For this review, take the finished solid that the model builds, in its own axes (mm). A direction names the side the tool comes from. Round coordinates to 2 decimals unless told otherwise and drop trailing zeros. Write each loop counter-clockwise with the first axis right and the second up, starting at its lowest first coordinate (ties: lowest second). Pieces come first, ordered by that corner, then holes. Notation, with made-up numbers: M 56.25,78 L 83.25,78 A23 cw 83.25,113 Z; hole C 31.25,24 d8. An arc over 180 degrees is marked long. Answer in a Markdown table with one row per item.
Autodesk Fusion 360 part; units mm, degrees
sketch "Sketch1" plane through (0, 0, 0) normal (0, 0, 1) x (1, 0, 0)
  line L0 (0, 0) -> (120, 0)
  line L1 (120, 0) -> (120, 50)
  line L2 (120, 50) -> (0, 50)
  line L3 (0, 50) -> (0, 0)
  line L4 (16.75, 41.3333) -> (103.25, 41.3333)
  line L5 (103.25, 41.3333) -> (103.25, 29.3333)
  line L6 (103.25, 29.3333) -> (16.75, 29.3333)
  line L7 (16.75, 29.3333) -> (16.75, 41.3333)
  line L8 (16.75, 20.6667) -> (103.25, 20.6667)
  line L9 (103.25, 20.6667) -> (103.25, 8.6667)
  line L10 (103.25, 8.6667) -> (16.75, 8.6667)
  line L11 (16.75, 8.6667) -> (16.75, 20.6667)
  line L12 (103.25, 35.3656) -> (120, 35.3656) construction
  line L13 (0, 36) -> (16.75, 36) construction
  line L14 (16.75, 14.6667) -> (0, 14.6667) construction
  line L15 (103.25, 14.6667) -> (120, 14.6667) construction
  line L16 (54.6731, 50) -> (54.6731, 41.3333) construction
  line L17 (54.6731, 29.3333) -> (54.6731, 20.6667) construction
  line L18 (56.6135, 8.6667) -> (56.6135, 0) construction
  dimension "d1" = 120
  dimension "d2" = 50
  dimension "d3" = 86.5
  dimension "d4" = 12
  dimension "d6" = 86.5
  dimension "d7" = 12
extrude "Extrude1" add sketch "Sketch1" along normal blind 2
sketch "Sketch2" plane through (0, 0, 2) normal (0, 0, 1) x (-1, 0, 0)
  line L0 (-103.25, -8.6667) -> (-16.75, -8.6667)
  line L1 (-16.75, -8.6667) -> (-16.75, -20.6667)
  line L2 (-16.75, -20.6667) -> (-103.25, -20.6667)
  line L3 (-103.25, -20.6667) -> (-103.25, -8.6667)
  line L4 (-103.25, -29.3333) -> (-16.75, -29.3333)
  line L5 (-16.75, -29.3333) -> (-16.75, -41.3333)
  line L6 (-16.75, -41.3333) -> (-103.25, -41.3333)
  line L7 (-103.25, -41.3333) -> (-103.25, -29.3333)
  line L8 (0, -50) -> (0, 0)
  line L9 (0, 0) -> (-120, 0)
  line L10 (-120, 0) -> (-120, -50)
  line L11 (-120, -50) -> (0, -50)
  line L12 (-2, -48) -> (-118, -48)
  line L13 (-118, -48) -> (-118, -2)
  line L14 (-118, -2) -> (-2, -2)
  line L15 (-2, -2) -> (-2, -48)
  dimension "d10" = 2
  dimension "d11" = 2
  dimension "d12" = 2
  dimension "d13" = 2
extrude "Extrude2" add sketch "Sketch2" along normal blind 50 contours L8 L9 L10 L11
sketch "Sketch3" plane through (0, 0, 0) normal (-1, 0, 0) x (0, -1, 0)
  line L0 (-50, 0) -> (0, 0)
  line L1 (0, 0) -> (0, 52)
  line L2 (0, 52) -> (-50, 52)
  line L3 (-50, 52) -> (-50, 0)
  line L4 (-31, 47) -> (-19, 47)
  line L5 (-19, 47) -> (-19, 42)
  line L6 (-19, 42) -> (-31, 42)
  line L7 (-31, 42) -> (-31, 47)
  line L8 (-31, 44.5) -> (-50, 44.5) construction
  line L9 (-40.8681, 44.5) -> (-40.5, 44.5) construction
  line L10 (-19, 44.5) -> (0, 44.5) construction
  dimension "d16" = 12
  dimension "d17" = 5
  dimension "d18" = 5
extrude "Extrude3" cut sketch "Sketch3" against normal blind 10 contours L4 L5 L6 L7
Q1. Take a section at C-C (z = 32.5). State the section outline as (x, y) points.
Found:
| item | result |
|---|---|
| outline | M 0,0 L 120,0 L 120,50 L 0,50 Z; hole M 2,2 L 118,2 L 118,48 L 2,48 Z |
Q2. Take a section at D-D (z = 45). State the section outline as (x, y) points, then the cut area to 3 significant figures.
Found:
| item | result |
|---|---|
| outline | M 0,0 L 120,0 L 120,50 L 0,50 L 0,31 L 2,31 L 2,48 L 118,48 L 118,2 L 2,2 L 2,19 L 0,19 Z |
| area | 640 mm² |
Q3. Take a section at B-B (y = 34.5). State the section outline as (x, z) points, then the cut area to 3 significant figures.
Found:
| item | result |
|---|---|
| outline | M 0,0 L 16.75,0 L 16.75,2 L 2,2 L 2,52 L 0,52 Z; M 103.25,0 L 120,0 L 120,52 L 118,52 L 118,2 L 103.25,2 Z |
| area | 267 mm² |
Q4. For probe 1 along X at (y, z) = (14.5, 22); probe 2 along Y at (x, z) = (93.5, 8); probe 3 along Z at (x, y) = (8, 38), list the stretches that pass through material, from the lowest coordinate up.
Found:
| item | result |
|---|---|
| probe 1 | 0 to 2, 118 to 120 |
| probe 2 | 0 to 2, 48 to 50 |
| probe 3 | 0 to 2 |
Q5. Machinability: for faces 4 (the face through (2, 25, 27)), 5 (the face through (61, 50, 26)), which of the approach directions +Z, -Z, +X, -X, +Y, -Y give a long, thin tool a straight path to every point of the face, cutting with its end or side? Answer none if there is none.
Found:
| item | result |
|---|---|
| face 4 | +Z |
| face 5 | +Z, -Z, +X, -X, +Y |
Q6. Mouldability with a two-part tool opening along X and no side actions: class faces 1 (the face through (59, 25, 0)), 2 (the face through (61, 2, 27)), 3 (the face through (120, 25, 26)) as +X half, -X half, draft (parallel to the pull), parting line (faces both ways), or undercut.
Found:
| item | result |
|---|---|
| face 1 | draft |
| face 2 | undercut |
| face 3 | +X half |
Q7. Take a section at A-A (x = 76.5). State the section outline as (y, z) points, then the cut area to 3 significant figures.
Found:
| item | result |
|---|---|
| outline | M 0,0 L 8.67,0 L 8.67,2 L 2,2 L 2,52 L 0,52 Z; M 20.67,0 L 29.33,0 L 29.33,2 L 20.67,2 Z; M 41.33,0 L 50,0 L 50,52 L 48,52 L 48,2 L 41.33,2 Z |
| area | 252 mm² |
